Here's how the part is built. I have some questions about the finished solid (model axes, mm). A direction names the side the tool comes from. Give positions to 0.01 mm unless a question says otherwise; leave off trailing zeros. Write each loop counter-clockwise with the first axis right and the second up, starting at its lowest first coordinate (ties: lowest second). Pieces come first, ordered by that corner, then holes. Notation, with made-up numbers: (51, -27) -> (96, -27) arc R32 ccw to (96, 5) -> close; hole circle Ø11 at (76, 34). An arc over 180 degrees is marked (long way). Use one line per item in the form item = value.
```python
from build123d import *

# Parameters (mm, degrees)
SKETCH_W        = 90
SKETCH_H        = 10
PAD_DEPTH       = 113
SKETCH001_R     = 2.25
SKETCH001_R_2   = 3.25
POCKET_DEPTH    = 10.001
SKETCH002_R     = 6
POCKET001_DEPTH = 4


with BuildPart() as part:
    # Sketch → Pad (new body)
    with BuildSketch(Plane.XY):
        Rectangle(SKETCH_W, SKETCH_H)
    extrude(amount=PAD_DEPTH)

    # Sketch001 → Pocket (cut, through all)
    with BuildSketch(Plane.XZ.offset(5)):
        with Locations((-30, 103)):
            Circle(SKETCH001_R)
        with Locations((30, 103)):
            Circle(SKETCH001_R)
        with Locations((28, 9)):
            Circle(SKETCH001_R)
        with Locations((-28, 9)):
            Circle(SKETCH001_R)
        with Locations((0, 82.5)):
            Circle(SKETCH001_R_2)
        with Locations((0, 30.5)):
            Circle(SKETCH001_R_2)
        with Locations((26, 56.5)):
            Circle(SKETCH001_R_2)
        with Locations((-26, 56.5)):
            Circle(SKETCH001_R_2)
    extrude(amount=-POCKET_DEPTH, mode=Mode.SUBTRACT)

    # Sketch002 → Pocket001 (cut)
    with BuildSketch(Plane.XZ.offset(5)):
        with Locations((0, 82.5)):
            Circle(SKETCH002_R)
    extrude(amount=-POCKET001_DEPTH, mode=Mode.SUBTRACT)


solid = part.part
```
Q1. I want a section at A-A, the plane z = 30.5. Write out the boundary of the cut face in (x, y).
Result set:
outline = (-45, -5) -> (-3.25, -5) -> (-3.25, 5) -> (-45, 5) -> close; (3.25, -5) -> (45, -5) -> (45, 5) -> (3.25, 5) -> close
Q2. Which directions (+Z, -Z, +X, -X, +Y, -Y) give clear straight access to the entire face, cutting with the end or side of a thin tool? Please do faces 5 (the face through (3, -1, 80)), 6 (the face through (-45, 0, 56)).
Result set:
face_5 = -Y
face_6 = +Z, -Z, -X, +Y, -Y
Q3. If we mould it in two halves opening along Z, with no side actions, what happens to faces 1 (the face through (-1, 0, 0)), 2 (the face through (-26.423, -0.07, 59.722)), 3 (the face through (-1, 0, 113)), 4 (the face through (45, 0, 56))? For each: +Z half, -Z half, draft (parallel to the pull), parting line (faces both ways), or undercut.
Result set:
face_1 = -Z half
face_2 = undercut
face_3 = +Z half
face_4 = draft
Q4. I want a section at B-B, the plane z = 9. Write out the boundary of the cut face in (x, y), and give its area (3 significant figures).
Result set:
outline = (-45, -5) -> (-30.25, -5) -> (-30.25, 5) -> (-45, 5) -> close; (-25.75, -5) -> (25.75, -5) -> (25.75, 5) -> (-25.75, 5) -> close; (30.25, -5) -> (45, -5) -> (45, 5) -> (30.25, 5) -> close
area = 810 mm2
Q5. I want a section at C-C, the plane y = 2.25. Count the separate pieces of the cut face and the enclosed holes in it, and give its area (3 significant figures).
Result set:
separate_pieces = 1
enclosed_holes = 8
area = 9,970 mm2
Q6. If I drill on line 1 along Z through (x, y) = (0, 0.55); line 2 along X through (y, z) = (-1, 59); line 3 along Z through (x, y) = (26, 2), over which ranges is the centre line in solid material (lowest first)? Write a range as from..to.
Result set:
line_1 = 0..27.25, 33.75..79.25, 85.75..113
line_2 = -45..-28.08, -23.92..23.92, 28.08..45
line_3 = 0..7.97, 10.03..53.25, 59.75..113
Q7. Will these pins go through, and if not, where does the flat tip stop? pin 1 Ø7.5 at (x, z) = (0, 82.5) entering from -Y; pin 2 Ø5 at (x, z) = (26, 56.5) entering from +Y.
Result set:
pin_1 = -1
pin_2 = through
